Input: dimensioned drawing with shaded views. Units: mm. Origin: part minimum x, y, z. Round coordinates to 2 decimals unless told otherwise and drop trailing zeros. Write each loop counter-clockwise with the first axis right and the second up, starting at its lowest first coordinate (ties: lowest second). Pieces come first, ordered by that corner, then holes. Notation, with made-up numbers: (-34.75, 22) -> (2.25, 22) arc R10 ccw to (2.25, 34) -> close; hole circle Ø6 at (23.25, 13.25). An arc over 180 degrees is marked (long way). Use one line per item in the form item = value. Start each with the question number.
1. Pin query (flat end, axial travel): pin 1 Ø0.6 at (x, y) = (103, 1.5) entering from +Z; pin 2 Ø1 at (x, y) = (46, 0.5) entering from +Z; pin 3 Ø1 at (y, z) = (1.5, 36) entering from -X; pin 4 Ø0.6 at (y, z) = (1, 42) entering from -X. Return the tip coordinate at first contact, or that it passes through.
2. Cut plane A-A, the plane z = 30. Return the cut outline in (x, y).
3. Cut plane C-C, the plane x = 61.5. Return the cut outline in (y, z), plus the area to 3 significant figures.
4. Line query: L1, parallel to X at y = 0.8, z = 33; L2, parallel to X at y = 1.8, z = 40.5; L3, parallel to Z at x = 36, y = 0.75. Output: solid intervals per line, ascending.
5. Cut plane B-B, the plane y = 1.45. Return the cut outline in (x, z), plus the area to 3 significant figures.
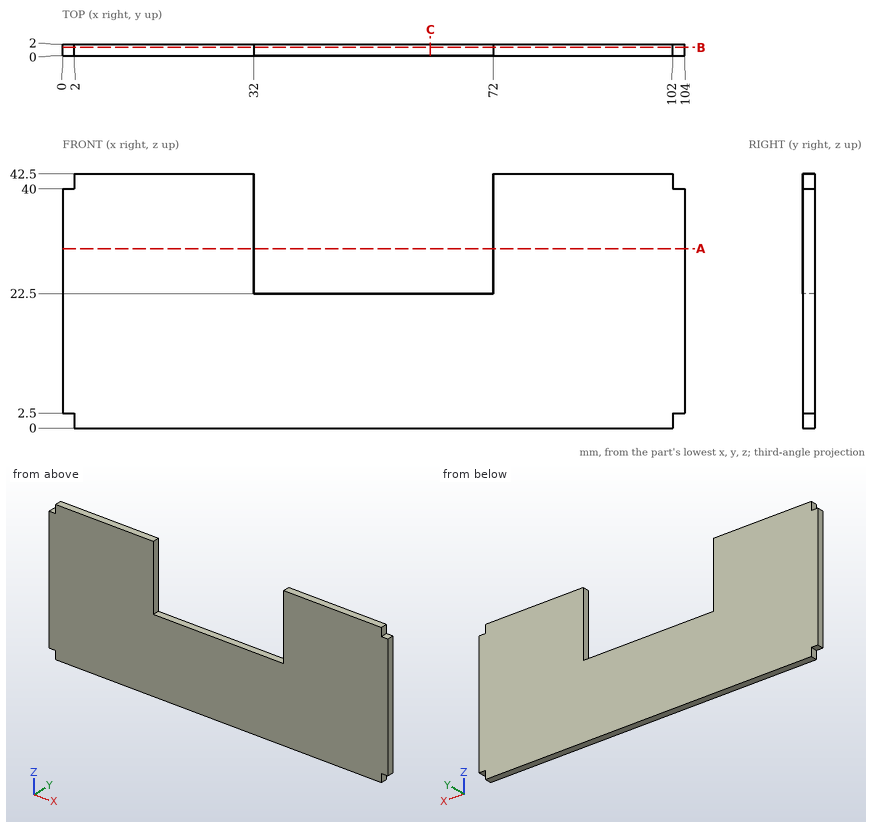
Outcome:
q1.pin_1 = 40
q1.pin_2 = 22.5
q1.pin_3 = 0
q1.pin_4 = 2
q2.outline = (0, 0) -> (32, 0) -> (32, 2) -> (0, 2) -> close; (72, 0) -> (104, 0) -> (104, 2) -> (72, 2) -> close
q3.outline = (0, 0) -> (2, 0) -> (2, 22.5) -> (0, 22.5) -> close
q3.area = 45.0 mm^2
q4.L1 = 0 to 32, 72 to 104
q4.L2 = 2 to 32, 72 to 102
q4.L3 = 0 to 22.5
q5.outline = (0, 2.5) -> (2, 2.5) -> (2, 0) -> (102, 0) -> (102, 2.5) -> (104, 2.5) -> (104, 40) -> (102, 40) -> (102, 42.5) -> (72, 42.5) -> (72, 22.5) -> (32, 22.5) -> (32, 42.5) -> (2, 42.5) -> (2, 40) -> (0, 40) -> close
q5.area = 3,600 mm^2
